```python
from build123d import *

# Parameters (mm, degrees)
F1_DEPTH = 25.4


with BuildPart() as f1:
    # F0 (on Front) → F1 (new body)
    with BuildSketch(Plane.XZ):
        Polygon((6.4789838679, 143.0610253916), (0, 190.1048020358), (-6.6051132214, 143.363907551), (0, 162.5912040472), align=None)
        Polygon((0, 162.5912040472), (-6.6051132214, 143.363907551), (-11.2874526005, 110.2294670761), (0, 127.4327933788), (10.8845930701, 111.0719821234), (6.4789838679, 143.0610253916), align=None)
        Polygon((-11.2874526005, 110.2294670761), (-6.6051132214, 143.363907551), (-25.3510719107, 88.7949556276), align=None)
        Polygon((23.2641081299, 92.464128984), (6.4789838679, 143.0610253916), (10.8845930701, 111.0719821234), align=None)
        Polygon((-16.1964657783, 75.4909759594), (-11.2874526005, 110.2294670761), (-25.3510719107, 88.7949556276), (-34.5284807194, 62.0797799271), align=None)
        Polygon((-34.5284807194, 62.0797799271), (-25.3510719107, 88.7949556276), (-50.5880084585, 50.3310727943), align=None)
        Polygon((23.2641081299, 92.464128984), (10.8845930701, 111.0719821234), (15.9783431129, 74.0863615106), (33.7067852385, 60.9858364417), align=None)
        Polygon((54.3591441951, 45.7246677317), (23.2641081299, 92.464128984), (33.7067852385, 60.9858364417), align=None)
        Polygon((-42.8858424978, 37.7517377794), (-34.5284807194, 62.0797799271), (-50.5880084585, 50.3310727943), (-63.1169358373, 31.2356016062), align=None)
        Polygon((-63.1169358373, 31.2356016062), (-50.5880084585, 50.3310727943), (-87.3659343428, 23.4253575589), align=None)
        Polygon((54.3591441951, 45.7246677317), (33.7067852385, 60.9858364417), (41.2983510128, 38.1019029624), (64.4518457344, 30.554161689), align=None)
        Polygon((83.1275046372, 24.4661372589), (54.3591441951, 45.7246677317), (64.4518457344, 30.554161689), align=None)
        Polygon((-72.7158875117, 16.6057374852), (-63.1169358373, 31.2356016062), (-87.3659343428, 23.4253575589), (-102.4342347336, 12.401804989), align=None)
        Polygon((-102.4342347336, 12.401804989), (-87.3659343428, 23.4253575589), (-136.5947303766, 7.5694898993), align=None)
        Polygon((83.1275046372, 24.4661372589), (64.4518457344, 30.554161689), (73.837026265, 16.4471421365), (98.7480565931, 12.92324866), align=None)
        Polygon((133.7063873813, 7.9780724792), (83.1275046372, 24.4661372589), (98.7480565931, 12.92324866), align=None)
        Polygon((-119.3864941597, 0), (-102.4342347336, 12.401804989), (-136.5947303766, 7.5694898993), (-160.0962430239, 0), (-145.7079445735, -4.2353132382), (-108.3147829025, -7.8024970817), align=None)
        Polygon((-160.0962430239, 0), (-136.5947303766, 7.5694898993), (-190.1048020358, 0), (-145.7079445735, -4.2353132382), align=None)
        Polygon((133.7063873813, 7.9780724792), (98.7480565931, 12.92324866), (116.2365972996, 0), (105.0231827748, -8.116504838), (143.1423881699, -4.4800588265), (158.1799685955, 0), align=None)
        Polygon((190.1048020358, 0), (133.7063873813, 7.9780724792), (158.1799685955, 0), (143.1423881699, -4.4800588265), align=None)
        Polygon((-64.3567517854, -28.1817016834), (-76.1863177081, -10.8674463087), (-108.3147829025, -7.8024970817), (-90.185094151, -20.5789180242), align=None)
        Polygon((-90.185094151, -20.5789180242), (-108.3147829025, -7.8024970817), (-145.7079445735, -4.2353132382), align=None)
        Polygon((105.0231827748, -8.116504838), (77.3257177694, -10.7587513145), (65.6897330033, -27.5550776524), (86.8962872603, -21.237132352), align=None)
        Polygon((143.1423881699, -4.4800588265), (105.0231827748, -8.116504838), (86.8962872603, -21.237132352), align=None)
        Polygon((-34.6929381596, -59.6855543086), (-43.7076647237, -34.2599292161), (-64.3567517854, -28.1817016834), (-50.3907510083, -48.6229338974), align=None)
        Polygon((-50.3907510083, -48.6229338974), (-64.3567517854, -28.1817016834), (-90.185094151, -20.5789180242), align=None)
        Polygon((65.6897330033, -27.5550776524), (42.0972347258, -34.58385337), (33.4121165087, -59.9500979433), (53.139639768, -45.6709024653), align=None)
        Polygon((86.8962872603, -21.237132352), (65.6897330033, -27.5550776524), (53.139639768, -45.6709024653), align=None)
        Polygon((-12.0666112155, -104.7157734591), (-16.6312789161, -72.4140332461), (-34.6929381596, -59.6855543086), (-25.9125275508, -84.4503019369), align=None)
        Polygon((-25.9125275508, -84.4503019369), (-34.6929381596, -59.6855543086), (-50.3907510083, -48.6229338974), align=None)
        Polygon((33.4121165087, -59.9500979433), (16.2104519289, -72.4010238832), (11.6420852362, -105.5718461452), (23.8011252741, -88.0204993073), align=None)
        Polygon((53.139639768, -45.6709024653), (33.4121165087, -59.9500979433), (23.8011252741, -88.0204993073), align=None)
        Polygon((-7.6525536308, -135.9517255008), (-12.0666112155, -104.7157734591), (-25.9125275508, -84.4503019369), align=None)
        Polygon((0, -122.3769783974), (-12.0666112155, -104.7157734591), (-7.6525536308, -135.9517255008), (0, -157.5354039669), (7.5039086249, -135.6190665407), (11.6420852362, -105.5718461452), align=None)
        Polygon((23.8011252741, -88.0204993073), (11.6420852362, -105.5718461452), (7.5039086249, -135.6190665407), align=None)
        Polygon((0, -157.5354039669), (-7.6525536308, -135.9517255008), (0, -190.1048020358), (7.5039086249, -135.6190665407), align=None)
        Polygon((-23.5345997346, 23.5628812437), (-20.5111412815, 44.9582983698), (-42.8858424978, 37.7517377794), (-48.9974841566, 19.9609229495), align=None)
        Polygon((-48.9974841566, 19.9609229495), (-42.8858424978, 37.7517377794), (-63.1169358373, 31.2356016062), (-72.7158875117, 16.6057374852), align=None)
        Polygon((-20.5111412815, 44.9582983698), (-16.1964657783, 75.4909759594), (-34.5284807194, 62.0797799271), (-42.8858424978, 37.7517377794), align=None)
        Polygon((-43.7076647237, -34.2599292161), (-51.1548930664, -13.2553613598), (-76.1863177081, -10.8674463087), (-64.3567517854, -28.1817016834), align=None)
        Polygon((-21.0818016053, -40.9200369363), (-24.6336619422, -15.7853990178), (-51.1548930664, -13.2553613598), (-43.7076647237, -34.2599292161), align=None)
        Polygon((-16.6312789161, -72.4140332461), (-21.0818016053, -40.9200369363), (-43.7076647237, -34.2599292161), (-34.6929381596, -59.6855543086), align=None)
        Polygon((42.0972347258, -34.58385337), (20.5339658906, -41.0080725688), (16.2104519289, -72.4010238832), (33.4121165087, -59.9500979433), align=None)
        Polygon((49.3406122431, -13.4284377447), (23.9993605016, -15.8459092755), (20.5339658906, -41.0080725688), (42.0972347258, -34.58385337), align=None)
        Polygon((33.7067852385, 60.9858364417), (15.9783431129, 74.0863615106), (19.9769714734, 45.0523982672), (41.2983510128, 38.1019029624), align=None)
        Polygon((41.2983510128, 38.1019029624), (19.9769714734, 45.0523982672), (22.9246777033, 23.6491603032), (47.2337087064, 20.2104251467), align=None)
        Polygon((64.4518457344, 30.554161689), (41.2983510128, 38.1019029624), (47.2337087064, 20.2104251467), (73.837026265, 16.4471421365), align=None)
        Polygon((77.3257177694, -10.7587513145), (49.3406122431, -13.4284377447), (42.0972347258, -34.58385337), (65.6897330033, -27.5550776524), align=None)
    extrude(amount=F1_DEPTH)


solid = f1.part
```
Check sheet for the modelled part. Datum: model origin and axes. Units: mm. A direction names the side the tool comes from. Coordinates: 2 decimals unless noted, no trailing zeros. Order: outer loops, then holes, each group sorted by start corner. A loop starts at its lowest first (then second) coordinate and runs counter-clockwise, first axis right, second up. Notation, with made-up numbers: (87.5, 33) -> (142.5, 33) arc R21 ccw to (142.5, 48) -> close; hole circle Ø2 at (-36, -5). An arc over 180 degrees is marked (long way). Write each question's results on one line, items separated by ' | '. Start each with the question number.
1) Section check B-B (x = -42). Enter the section's corners in (y, z), and give its area (3 significant figures).
2) Section check C-C (x = 159.5). Enter the section's corners in (y, z), and give its area (3 significant figures).
3) Section check D-D (z = -160.5). Enter the section's corners in (x, y).
4) Material ranges on line 1 along X through (y, z) = (-6.5, 95.5); line 2 along X through (y, z) = (-9.5, 130); line 3 along X through (y, z) = (-18.5, 112.5), recorded low to high.
5) Set-up check for faces 1 (the face through (-5.723, -12.522, 118.711)), 2 (the face through (-15.847, -12.522, 116.461)): record each of +Z, -Z, +X, -X, +Y, -Y from which the full face is reachable in a straight line by a thin tool's end or side.
6) Section check A-A (z = -35). Enter the section's corners in (x, y).
7) Depth check by flat-ended pin: pin 1 (1.5 mm diameter, centred on y = -14, z = -46, fed in from +X); pin 2 (12 mm diameter, centred on y = -8.5, z = 96.5, fed in from -X); pin 3 (10 mm diameter, centred on y = -8, z = 150.5, fed in from +X). Enter the tip coordinate at first touch or a pass-through.
8) Draft check along X on faces 3 (the face through (-70.57, -12.52, -34.4)), 4 (the face through (166.29, -12.52, -2.27)), 5 (the face through (5.9, -12.52, -113.86)), 6 (the face through (5.366, -12.522, 119.367)). Enter one of: pulls with the +X half, pulls with the -X half, needs draft (parallel to the pull), parting line crosses it, or undercut.
Checked values:
1) outline: (-25.4, -60.9) -> (0, -60.9) -> (0, -14.13) -> (-25.4, -14.13) -> close; (-25.4, 20.95) -> (0, 20.95) -> (0, 63.42) -> (-25.4, 63.42) -> close | area: 2,270 mm²
2) outline: (-25.4, -2.92) -> (0, -2.92) -> (0, 4.33) -> (-25.4, 4.33) -> close | area: 184 mm²
3) outline: (-4.18, -25.4) -> (4.08, -25.4) -> (4.08, 0) -> (-4.18, 0) -> close
4) line 1: -23.05 to -13.37, 13.03 to 22.26 | line 2: -11.2 to 10.81 | line 3: -17.21 to -9.8, 9.93 to 16.62
5) face 1: +Y, -Y | face 2: +Z, -X, +Y, -Y
6) outline: (-69.72, -25.4) -> (-21.92, -25.4) -> (-21.92, 0) -> (-69.72, 0) -> close; (21.36, -25.4) -> (67.88, -25.4) -> (67.88, 0) -> (21.36, 0) -> close
7) pin 1: x = 53.72 | pin 2: x = -24.77 | pin 3: x = 6.14
8) face 3: pulls with the -X half | face 4: pulls with the +X half | face 5: undercut | face 6: undercut
